Build history of the part. All positions in model axes, mm. Face numbers are marked on the shaded views. A direction names the side the tool comes from. Give positions to 0.01 mm unless a question says otherwise; leave off trailing zeros. Loops run counter-clockwise (first coordinate to the right, second up) from the corner with the lowest first, then second, coordinate; pieces in that order, holes last. Notation, with made-up numbers: M -23.75,45 L 14.25,45 A13 ccw 14.25,52 Z; hole C 75,17 d2. An arc over 180 degrees is marked long. Answer in a Markdown table with one row per item. Add a question column.
```python
from build123d import *

# Parameters (mm, degrees)
SKETCH1_W           = 230
SKETCH1_H           = 230
SKETCH1_W_2         = 200
SKETCH1_H_2         = 200
BOSS_EXTRUDE1_DEPTH = 30
SKETCH2_R           = 11
CUT_EXTRUDE3_DEPTH  = 206
SKETCH3_W           = 12.648408852
SKETCH3_H           = 30
BOSS_EXTRUDE2_DEPTH = 28
SKETCH4_W           = 33.277006623
SKETCH4_H           = 30
BOSS_EXTRUDE4_DEPTH = 41
SKETCH6_R           = 4
CUT_EXTRUDE4_DEPTH  = 218
SKETCH8_R           = 4.046690546
CUT_EXTRUDE6_DEPTH  = 280
CUT_EXTRUDE7_START  = -230
SKETCH9_R           = 11
CUT_EXTRUDE7_DEPTH  = 230
SKETCH11_W          = 19.776160892
SKETCH11_H          = 30
CUT_EXTRUDE8_DEPTH  = 41
SKETCH12_R          = 4
CUT_EXTRUDE9_DEPTH  = 264
SKETCH13_R          = 4
CUT_EXTRUDE10_DEPTH = 264
SKETCH15_W          = 8.223839108
SKETCH15_H          = 30
CUT_EXTRUDE11_DEPTH = 64
SKETCH16_W          = 6.512440182
SKETCH16_H          = 30
BOSS_EXTRUDE5_DEPTH = 40
SKETCH17_R          = 4
CUT_EXTRUDE12_DEPTH = 276


with BuildPart() as part:
    # Sketch1 → Boss-Extrude1 (new body)
    with BuildSketch(Plane(origin=(0, 0, 0), x_dir=(1, 0, 0), z_dir=(0, 1, 0))):
        Rectangle(SKETCH1_W, SKETCH1_H)
        Rectangle(SKETCH1_W_2, SKETCH1_H_2, mode=Mode.SUBTRACT)
    extrude(amount=BOSS_EXTRUDE1_DEPTH)

    # Sketch2 → Cut-Extrude3 (cut)
    with BuildSketch(Plane(origin=(115, 0, 0), x_dir=(0, 0, -1), z_dir=(1, 0, 0))):
        with Locations((0, 15)):
            Circle(SKETCH2_R)
    extrude(amount=-CUT_EXTRUDE3_DEPTH, mode=Mode.SUBTRACT)

    # Sketch3 → Boss-Extrude2 (add)
    with BuildSketch(Plane(origin=(115, 0, 0), x_dir=(0, 0, -1), z_dir=(1, 0, 0))):
        with Locations((26.610788675, 15)):
            Rectangle(SKETCH3_W, SKETCH3_H)
    extrude(amount=BOSS_EXTRUDE2_DEPTH)

    # Sketch4 → Boss-Extrude4 (add)
    with BuildSketch(Plane.XY.offset(-20.286584249)):
        with Locations((126.361496689, 15)):
            Rectangle(SKETCH4_W, SKETCH4_H)
    extrude(amount=BOSS_EXTRUDE4_DEPTH)

    # Sketch6 → Cut-Extrude4 (cut)
    with BuildSketch(Plane.ZY.offset(115)):
        with Locations((0, 15)):
            Circle(SKETCH6_R)
    extrude(amount=-CUT_EXTRUDE4_DEPTH, mode=Mode.SUBTRACT)

    # Sketch8 → Cut-Extrude6 (cut)
    with BuildSketch(Plane.XY.offset(115)):
        with Locations((0, 16.175919114)):
            Circle(SKETCH8_R)
    extrude(amount=-CUT_EXTRUDE6_DEPTH, mode=Mode.SUBTRACT)

    # Sketch9 → Cut-Extrude7 (cut)
    with BuildSketch(Plane.ZY.offset(115).offset(CUT_EXTRUDE7_START)):
        with Locations((0, 15)):
            Circle(SKETCH9_R)
    extrude(amount=CUT_EXTRUDE7_DEPTH, mode=Mode.SUBTRACT)

    # Sketch11 → Cut-Extrude8 (cut)
    with BuildSketch(Plane.XY.offset(20.713415751)):
        with Locations((124.888080446, 15)):
            Rectangle(SKETCH11_W, SKETCH11_H)
    extrude(amount=-CUT_EXTRUDE8_DEPTH, mode=Mode.SUBTRACT)

    # Sketch12 → Cut-Extrude9 (cut)
    with BuildSketch(Plane.ZY.offset(115)):
        with Locations((0, 15)):
            Circle(SKETCH12_R)
    extrude(amount=-CUT_EXTRUDE9_DEPTH, mode=Mode.SUBTRACT)

    # Sketch13 → Cut-Extrude10 (cut)
    with BuildSketch(Plane(origin=(0, 30, 0), x_dir=(1, 0, 0), z_dir=(0, 1, 0))):
        with Locations(Location((106.851068212, -106.17718303, 0), (0, 0, 270))):
            Circle(SKETCH13_R)
    extrude(amount=-CUT_EXTRUDE10_DEPTH, mode=Mode.SUBTRACT)

    # Sketch15 → Cut-Extrude11 (cut)
    with BuildSketch(Plane.XY.offset(20.713415751)):
        with Locations((138.888080446, 15)):
            Rectangle(SKETCH15_W, SKETCH15_H)
    extrude(amount=-CUT_EXTRUDE11_DEPTH, mode=Mode.SUBTRACT)

    # Sketch16 → Boss-Extrude5 (add)
    with BuildSketch(Plane.XY.offset(-20.286584249)):
        with Locations((131.519940801, 15)):
            Rectangle(SKETCH16_W, SKETCH16_H)
    extrude(amount=BOSS_EXTRUDE5_DEPTH)

    # Sketch17 → Cut-Extrude12 (cut)
    with BuildSketch(Plane.ZY.offset(115)):
        with Locations((0, 15)):
            Circle(SKETCH17_R)
    extrude(amount=-CUT_EXTRUDE12_DEPTH, mode=Mode.SUBTRACT)


solid = part.part
```
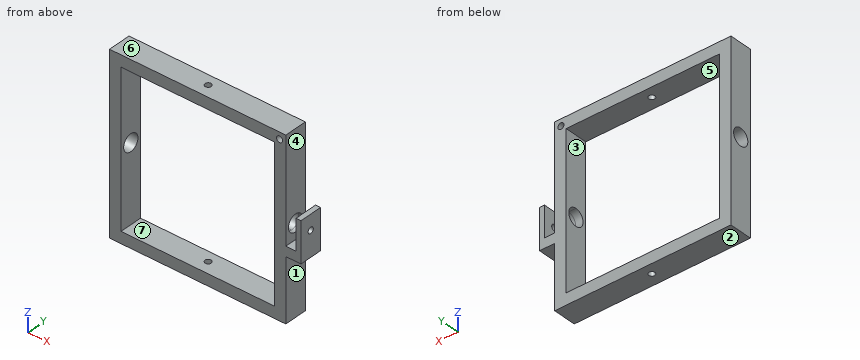
(1) Pull direction Z, two halves, no side cores. Call the marked faces 4, 5, 6 and 7: +Z half, -Z half, draft (parallel to the pull), parting line (faces both ways), or undercut.
(2) Wall check: line 1 (Z direction, x = -64, y = 24); line 2 (Y direction, x = 132.75, z = 0); line 3 (Y direction, x = 110.95, z = 0). Give the ranges that are in metal, low to high.
(3) Slice it at B-B, the plane z = 0. Give the cut face in (x, y), then the cut area to 3 significant figures.
(4) Pin check, flat tips, straight feed: pin 1 (6.5 mm diameter, centred on x = 124, y = 18, fed in from +Z); pin 2 (10.5 mm diameter, centred on y = 15, z = 0, fed in from +X); pin 3 (9 mm diameter, centred on y = 10, z = -88.5, fed in from +X); pin 4 (5 mm diameter, centred on x = 0, y = 16.18, fed in from -Z). Stop position of each tip, or through.
(5) Slice it at A-A, the plane x = -20. Give the cut face in (y, z), then the cut area to 3 significant figures.
(6) Tool access for the marked faces 1, 2 and 3: list every direction of +Z, -Z, +X, -X, +Y, -Y with a clear straight run to the whole face (end or side of a thin tool).
Solution:
| question | item | result |
|---|---|---|
| 1 | face 4 | draft |
| 1 | face 5 | undercut |
| 1 | face 6 | +Z half |
| 1 | face 7 | undercut |
| 2 | line 1 | -115 to -100, 100 to 115 |
| 2 | line 2 | 0 to 11, 19 to 30 |
| 2 | line 3 | 0 to 4, 26 to 30 |
| 3 | outline | M -115,0 L -100,0 L -100,4 L -115,4 Z; M -115,26 L -100,26 L -100,30 L -115,30 Z; M 100,0 L 115,0 L 115,4 L 100,4 Z; M 100,26 L 115,26 L 115,30 L 100,30 Z; M 128.26,0 L 134.78,0 L 134.78,11 L 128.26,11 Z; M 128.26,19 L 134.78,19 L 134.78,30 L 128.26,30 Z |
| 3 | area | 383 mm^2 |
| 4 | pin 1 | z = -20.29 |
| 4 | pin 2 | x = 134.78 |
| 4 | pin 3 | x = 115 |
| 4 | pin 4 | through |
| 5 | outline | M 0,-115 L 30,-115 L 30,-100 L 0,-100 Z; M 0,100 L 30,100 L 30,115 L 0,115 Z |
| 5 | area | 900 mm^2 |
| 6 | face 1 | -Z, +X, +Y, -Y |
| 6 | face 2 | -Z, +X, -X, +Y, -Y |
| 6 | face 3 | +Y, -Y |
